The listing builds one solid part. Answer for the finished solid, in the listing's coordinates (mm). Face numbers are marked on the shaded views. Round coordinates to 2 decimals unless told otherwise and drop trailing zeros. Loops run counter-clockwise (first coordinate to the right, second up) from the corner with the lowest first, then second, coordinate; pieces in that order, holes last. Notation, with made-up numbers: (7.5, -2.5) -> (36.5, -2.5) arc R20 cw to (36.5, 9.5) -> close; hole circle Ø5 at (-26.75, 0). An arc over 180 degrees is marked (long way). One line per question, with ' | ' between items.
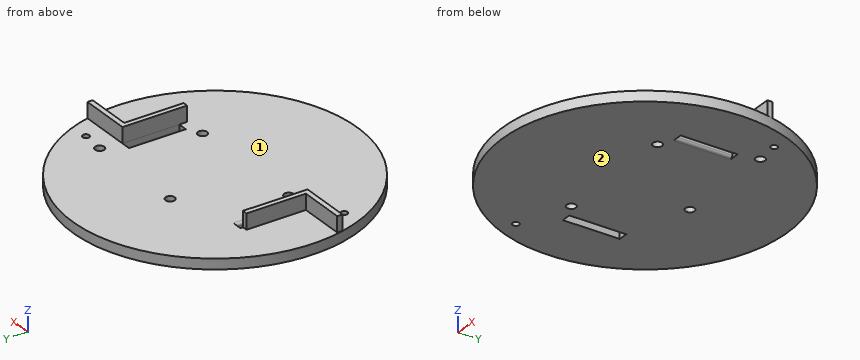
from build123d import *

# Parameters (mm, degrees)
SKETCH_R        = 55
PAD_DEPTH       = 4
SKETCH002_R     = 1.8
POCKET_DEPTH    = 5
PAD001_DEPTH    = 6
SKETCH003_R     = 1.3
POCKET001_DEPTH = 5
SKETCH004_W     = 3
SKETCH004_H     = 22
POCKET002_DEPTH = 5
FILLET_R        = 1
FILLET001_R     = 1
FILLET002_R     = 1
FILLET003_R     = 1


with BuildPart() as part:
    # Sketch → Pad (new body)
    with BuildSketch(Plane.XY):
        Circle(SKETCH_R)
    extrude(amount=PAD_DEPTH)

    # Sketch002 → Pocket (cut)
    with BuildSketch(Plane.XY.offset(4)):
        with Locations((-24.5, -11.840143)):
            Circle(SKETCH002_R)
        with Locations((24.5, -11.840143)):
            Circle(SKETCH002_R)
        with Locations((-5, 20.774952)):
            Circle(SKETCH002_R)
        with Locations((35, 20.774952)):
            Circle(SKETCH002_R)
    extrude(amount=-POCKET_DEPTH, mode=Mode.SUBTRACT)

    # Sketch001 (on Face3 of Pad) → Pad001 (join)
    with BuildSketch(Plane.XY.offset(4)):
        Polygon((33.500008, 0), (33.500008, 13), (53.345406, 13), (53.345406, 11), (35.5, 11), (35.5, -0.005684), (35.5, -12), (33.500008, -12), align=None)
        Polygon((-33.5, 0), (-33.5, -13), (-53.293575, -13), (-53.293575, -11), (-35.5, -11), (-35.5, 0.001212), (-35.5, 12), (-33.5, 12), align=None)
    extrude(amount=PAD001_DEPTH)

    # Sketch003 (on Face3 of Pad001) → Pocket001 (cut)
    with BuildSketch(Plane.XY.offset(4)):
        with Locations((-44, -20)):
            Circle(SKETCH003_R)
        with Locations((44, 20)):
            Circle(SKETCH003_R)
    extrude(amount=-POCKET001_DEPTH, mode=Mode.SUBTRACT)

    # Sketch004 → Pocket002 (cut)
    with BuildSketch(Plane.XY.offset(4)):
        with Locations((32, 2)):
            Rectangle(SKETCH004_W, SKETCH004_H)
    pocket002 = extrude(amount=-POCKET002_DEPTH, mode=Mode.SUBTRACT)

    # Mirrored: Pocket002 across Sketch004 V_Axis
    add(pocket002.mirror(Plane(origin=(0, 0, 4), x_dir=(0, 0, 1), z_dir=(1, 0, 0))), mode=Mode.SUBTRACT)

    # Fillet
    fillet_edges = [part.edges().sort_by_distance(p)[0] for p in [
        (30.5, 2, 4),
    ]]
    fillet(fillet_edges, radius=FILLET_R)

    # Fillet001
    fillet001_edges = [part.edges().sort_by_distance(p)[0] for p in [
        (-30.5, 2, 4),
    ]]
    fillet(fillet001_edges, radius=FILLET001_R)

    # Fillet002
    fillet002_edges = [part.edges().sort_by_distance(p)[0] for p in [
        (-30.5, 2, 0),
    ]]
    fillet(fillet002_edges, radius=FILLET002_R)

    # Fillet003
    fillet003_edges = [part.edges().sort_by_distance(p)[0] for p in [
        (30.5, 2, 0),
    ]]
    fillet(fillet003_edges, radius=FILLET003_R)


solid = part.part
Q1. For a pull along X with two mould halves and no side action, classify the marked faces 1 and 2 as pulls with the +X half, pulls with the -X half, needs draft (parallel to the pull), parting line crosses it, or undercut.
Numbers:
face 1: undercut | face 2: needs draft
Q2. Find the intervals of material crossed by line 1 (X direction, y = 1, z = 8.5); line 2 (Z direction, x = 24.5, y = -44.5); line 3 (Y direction, x = 44, z = 2.6), in increasing order. Write a range as from..to.
Numbers:
line 1: -35.5..-33.5, 33.5..35.5 | line 2: 0..4 | line 3: -33..18.7, 21.3..33
Q3. A cutting plane is placed at C-C on x = -44. Give the vertices of the cut face in (y, z).
Numbers:
outline: (-33, 0) -> (-21.3, 0) -> (-21.3, 4) -> (-33, 4) -> close; (-18.7, 0) -> (33, 0) -> (33, 4) -> (-11, 4) -> (-11, 10) -> (-13, 10) -> (-13, 4) -> (-18.7, 4) -> close
Q4. A cutting plane is placed at B-B on y = -20. Give the vertices of the cut face in (x, z), plus the area to 3 significant figures.
Numbers:
outline: (-51.23, 0) -> (-45.3, 0) -> (-45.3, 4) -> (-51.23, 4) -> close; (-42.7, 0) -> (51.23, 0) -> (51.23, 4) -> (-42.7, 4) -> close | area: 399 mm^2
Q5. A cutting plane is placed at D-D on y = 2. Give the number of separate pieces and of enclosed holes in the cut face, plus the area to 3 significant figures.
Numbers:
separate pieces: 3 | enclosed holes: 0 | area: 439 mm^2
Q6. Given pin 1 Ø4 at (x, y) = (35, 20.77) entering from +Z; pin 2 Ø1.8 at (y, z) = (-0.5, 7.5) entering from -X; pin 3 Ø1 at (y, z) = (27.5, 2.5) entering from +X; pin 4 Ø1.6 at (x, y) = (44, 20) entering from -Z, each flat-ended and moving along its own axis, determine where each tip first touches the part or whether it passes through.
Numbers:
pin 1: z = 4 | pin 2: x = -35.5 | pin 3: x = 47.92 | pin 4: through
Q7. A cutting plane is placed at A-A on z = 6. Give the vertices of the cut face in (x, y).
Numbers:
outline: (-53.29, -13) -> (-33.5, -13) -> (-33.5, 12) -> (-35.5, 12) -> (-35.5, -11) -> (-53.29, -11) -> close; (33.5, -12) -> (35.5, -12) -> (35.5, 11) -> (53.35, 11) -> (53.35, 13) -> (33.5, 13) -> close
